The model under review builds one solid part; all positions refer to its coordinate system, in mm. A direction names the side the tool comes from. Coordinates: 2 decimals unless noted, no trailing zeros. Return JSON: item names as keys, results as strings.
```python
from build123d import *

# Parameters (mm, degrees)
SKETCH1_R               = 47.5
BOSS_EXTRUDE1_DEPTH     = 13
SKETCH2_R               = 33
CUT_EXTRUDE1_DEPTH      = 2.5
CUT_EXTRUDE2_START      = -2.5
SKETCH3_R               = 33
CUT_EXTRUDE2_DEPTH      = 2.5
SKETCH4_R               = 16
BOSS_EXTRUDE2_DEPTH     = 7.5
BOSS_EXTRUDE3_START     = 7.5
SKETCH5_R               = 16
BOSS_EXTRUDE3_DEPTH     = 7.5
SKETCH9_R               = 8
CUT_EXTRUDE3_DEPTH      = 72.003521039
FILLET1_R               = 1
FILLET2_R               = 1
CUT_EXTRUDE5_DEPTH      = 27
CUT_EXTRUDE5_DEPTH_BACK = 17
SKETCH13_W              = 5
SKETCH13_H              = 4.917634469
FILLET3_R               = 1
FILLET4_R               = 1


with BuildPart() as part:
    # Sketch1 → Boss-Extrude1 (new body)
    with BuildSketch(Plane.XY):
        with Locations(Location((0, 0, 0), (0, 0, 180))):
            Circle(SKETCH1_R)
    extrude(amount=BOSS_EXTRUDE1_DEPTH)

    # Sketch2 → Cut-Extrude1 (cut)
    with BuildSketch(Plane.XY.offset(13)):
        Circle(SKETCH2_R)
    extrude(amount=-CUT_EXTRUDE1_DEPTH, mode=Mode.SUBTRACT)

    # Sketch3 → Cut-Extrude2 (cut)
    with BuildSketch(Plane(origin=(0, 0, 0), x_dir=(-1, 0, 0), z_dir=(0, 0, -1)).offset(CUT_EXTRUDE2_START)):
        with Locations(Location((0, 0, 0), (0, 0, 180))):
            Circle(SKETCH3_R)
    extrude(amount=CUT_EXTRUDE2_DEPTH, mode=Mode.SUBTRACT)

    # Sketch4 → Boss-Extrude2 (add)
    with BuildSketch(Plane(origin=(0, 0, 2.5), x_dir=(-1, 0, 0), z_dir=(0, 0, -1))):
        Circle(SKETCH4_R)
    extrude(amount=BOSS_EXTRUDE2_DEPTH)

    # Sketch5 → Boss-Extrude3 (add)
    with BuildSketch(Plane.XY.offset(10.5).offset(BOSS_EXTRUDE3_START)):
        with Locations(Location((0, 0, 0), (0, 0, 180))):
            Circle(SKETCH5_R)
    extrude(amount=-BOSS_EXTRUDE3_DEPTH)

    # Sketch9 → Cut-Extrude3 (cut, through all)
    with BuildSketch(Plane(origin=(0, 0, -5), x_dir=(-1, 0, 0), z_dir=(0, 0, -1))):
        Circle(SKETCH9_R)
    extrude(amount=-CUT_EXTRUDE3_DEPTH, mode=Mode.SUBTRACT)

    # Fillet1
    fillet1_edges = [part.edges().sort_by_distance(p)[0] for p in [
        (16, 0, 2.5),
    ]]
    fillet(fillet1_edges, radius=FILLET1_R)

    # Fillet2
    fillet2_edges = [part.edges().sort_by_distance(p)[0] for p in [
        (16, 0, 10.5),
    ]]
    fillet(fillet2_edges, radius=FILLET2_R)

    # Sketch12 → Cut-Revolve1 (revolve, cut)
    with BuildSketch(Plane(origin=(0, 0, 0), x_dir=(0, 0, -1), z_dir=(1, 0, 0)), mode=Mode.PRIVATE) as cut_revolve1_sk:
        Polygon((-10.5, 47.5), (-8.505134927, 33), (-4.459991863, 33), (-2.40344568, 47.5), align=None)
    revolve(cut_revolve1_sk.sketch.rotate(Axis((0, 0, 31.244121173), (0, 0, -1)), 270), axis=Axis((0, 0, 31.244121173), (0, 0, -1)), mode=Mode.SUBTRACT)

    # Sketch13 → Cut-Extrude5 (cut, two sides: drawn at the far end of the back side and taken through both)
    with BuildSketch(Plane.XY.offset(-CUT_EXTRUDE5_DEPTH_BACK)):
        with Locations((-0.093134084, 8.041182766)):
            Rectangle(SKETCH13_W, SKETCH13_H)
    extrude(amount=CUT_EXTRUDE5_DEPTH + CUT_EXTRUDE5_DEPTH_BACK, mode=Mode.SUBTRACT)

    # Fillet3
    fillet3_edges = [part.edges().sort_by_distance(p)[0] for p in [
        (-33, 0, 2.5),
    ]]
    fillet(fillet3_edges, radius=FILLET3_R)

    # Fillet4
    fillet4_edges = [part.edges().sort_by_distance(p)[0] for p in [
        (-33, 0, 10.5),
    ]]
    fillet(fillet4_edges, radius=FILLET4_R)


solid = part.part
```
1. Insertion check: pin 1 Ø12 at (x, z) = (-8.5, 14) entering from +Y; pin 2 Ø1.5 at (x, z) = (4.5, 12.5) entering from +Y; pin 3 Ø1 at (x, y) = (5.5, -21.5) entering from +Z. Each pin has a flat end and moves straight along its axis. Give the tip position at first contact, or say it passes through.
Check values:
{"pin 1": "y = 47.43", "pin 2": "y = 47.35", "pin 3": "z = 10.5"}
2. The part is to be moulded in two halves that separate along Y. For faces 1 (the face through (3.8, 7.3, -5)), 2 (the face through (10.3, 46.37, 11.73)), 3 (the face through (0, 10.5, 6)), say which applies: released by +Y, released by -Y, zero draft, split by the parting line, or undercut.
Check values:
{"face 1": "zero draft", "face 2": "split by the parting line", "face 3": "undercut"}
3. Machinability: for faces 4 (the face through (3.47, -15.62, -1.7)), 5 (the face through (2.407, 9, 6)), 6 (the face through (-32.34, 10.18, 4.33)), which of the approach directions +Z, -Z, +X, -X, +Y, -Y give a long, thin tool a straight path to every point of the face, cutting with its end or side? Answer none if there is none.
Check values:
{"face 4": "-Z", "face 5": "+Z, -Z", "face 6": "none"}
4. To check wall thickness, follow line 1 (Y direction, x = 0, z = 12.6); line 2 (Z direction, x = -17, y = 24); line 3 (Y direction, x = 1.5, z = 11.25). State the ranges of each line that lie inside material, in increasing order.
Check values:
{"line 1": "-47.5 to -33, -16 to -8, 10.5 to 16, 33 to 47.5", "line 2": "2.5 to 10.5", "line 3": "-47.48 to -32.93, -15.96 to -7.86, 10.5 to 15.96, 32.93 to 47.48"}
